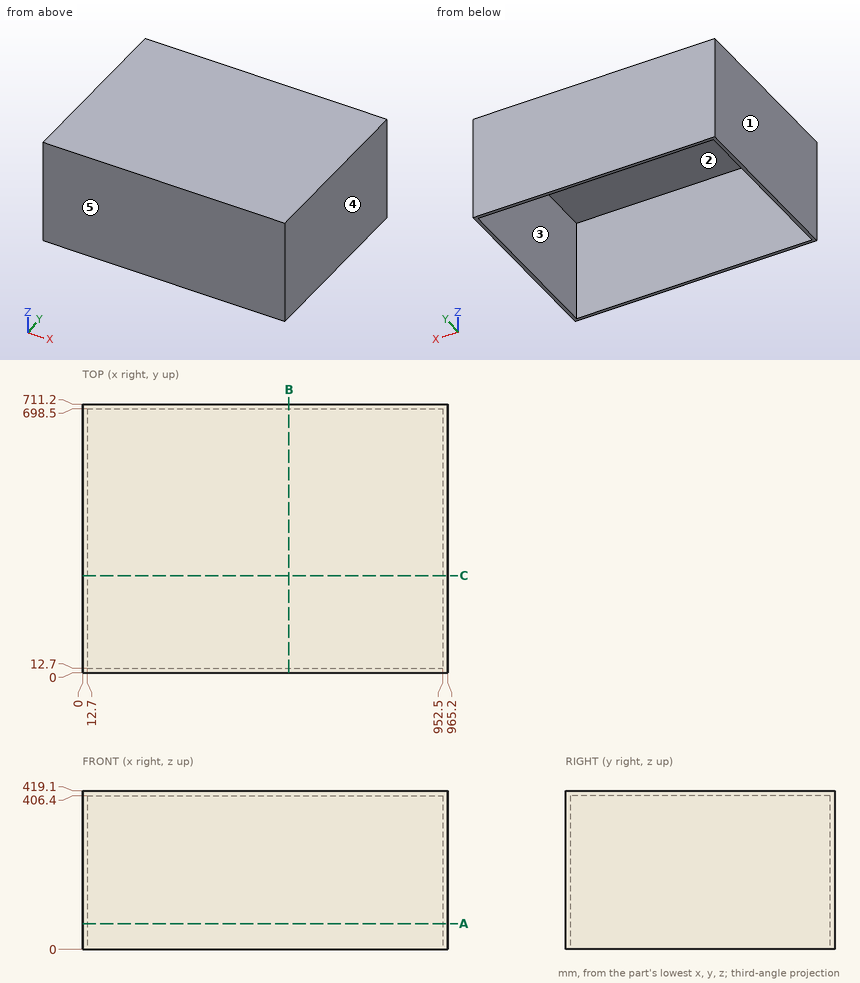
Can you work these out from the drawing? Everything is in mm from the part's minimum corner. A direction names the side the tool comes from. Give positions to 0.01 mm unless a question says otherwise; leave off trailing zeros. Order: outer loops, then holes, each group sorted by start corner. A loop starts at its lowest first (then second) coordinate and runs counter-clockwise, first axis right, second up. Notation, with made-up numbers: M 62,-34.5 L 82,-34.5 A12 cw 82,-30.5 Z; hole C -23.5,-16 d8. An arc over 180 degrees is marked long. One line per question, with ' | ' between items.
1. I want a section at A-A (z = 68). List the corners of the cut face in (x, y) for me.
Results:
outline: M 0,0 L 965.2,0 L 965.2,711.2 L 0,711.2 Z; hole M 12.7,12.7 L 952.5,12.7 L 952.5,698.5 L 12.7,698.5 Z
2. I want a section at C-C (y = 257.5). List the corners of the cut face in (x, z) for me.
Results:
outline: M 0,0 L 12.7,0 L 12.7,406.4 L 952.5,406.4 L 952.5,0 L 965.2,0 L 965.2,419.1 L 0,419.1 Z
3. I want a section at B-B (x = 546). List the corners of the cut face in (y, z) for me.
Results:
outline: M 0,0 L 12.7,0 L 12.7,406.4 L 698.5,406.4 L 698.5,0 L 711.2,0 L 711.2,419.1 L 0,419.1 Z
4. I'm going to push flat-ended pins straight in: pin 1 (1.5 mm diameter, centred on x = 143.5, y = 497.5, fed in from -Z); pin 2 (12 mm diameter, centred on x = 371.5, z = 248.5, fed in from -Y). Where does each tip first touch, or does it pass through?
Results:
pin 1: z = 406.4 | pin 2: y = 0
5. For the marked faces 1 and 2, which set-ups out of +Z, -Z, +X, -X, +Y, -Y let a thin tool reach every point of the face, with its end or its side?
Results:
face 1: +Z, -Z, -X, +Y, -Y | face 2: -Z
6. If I drill on line 1 (X direction, y = 260.5, z = 316.5); line 2 (Y direction, x = 640, z = 347.5); line 3 (Z direction, x = 285, y = 601), over which ranges is the centre line in solid material (lowest first)?
Results:
line 1: 0 to 12.7, 952.5 to 965.2 | line 2: 0 to 12.7, 698.5 to 711.2 | line 3: 406.4 to 419.1
7. We'd pull the mould along X, two halves only. Please class the marked faces 3, 4 and 5: +X half, -X half, draft (parallel to the pull), parting line (faces both ways), or undercut.
Results:
face 3: undercut | face 4: +X half | face 5: draft
